from build123d import *

# Parameters (mm, degrees)
F2_R     = 2.6
F3_DEPTH = 6
F4_R     = 4
F5_DEPTH = 28.401


with BuildPart() as f1:
    # F0 (on Front) → F1 (revolve)
    with BuildSketch(Plane.XZ):
        Polygon((48.080009, 8), (48.080009, 18.5), (21.681081, 18.262167), (21.681081, 28.4), (15.681081, 28.4), (15.681081, 8), align=None)
    revolve(axis=Axis((22.226226, 0, 0), (-1, 0, 0)))

    # F2 (on face) → F3 (cut)
    with BuildSketch(Plane.YZ.offset(21.681081)):
        with Locations((-23.400001, 0)):
            Circle(F2_R)
        with Locations((-11.7, -20.264995)):
            Circle(F2_R)
        with Locations((11.7, -20.264995)):
            Circle(F2_R)
        with Locations((23.400001, 0)):
            Circle(F2_R)
        with Locations((11.7, 20.264995)):
            Circle(F2_R)
        with Locations((-11.7, 20.264995)):
            Circle(F2_R)
    extrude(amount=-F3_DEPTH, mode=Mode.SUBTRACT)

    # F4 (on Front) → F5 (cut, through all)
    with BuildSketch(Plane.XZ):
        with Locations((37.880009, 0)):
            Circle(F4_R)
    extrude(amount=-F5_DEPTH, mode=Mode.SUBTRACT)


solid = f1.part
Verification items for the finished model (mm, model axes). A direction names the side the tool comes from. Coordinates: 2 decimals unless noted, no trailing zeros. Write each loop counter-clockwise with the first axis right and the second up, starting at its lowest first coordinate (ties: lowest second). Pieces come first, ordered by that corner, then holes. Notation, with made-up numbers: (70, 86.25) -> (85, 86.25) arc R18 cw to (85, 97.25) -> close; hole circle Ø8 at (-37, 88.5). An arc over 180 degrees is marked (long way). One line per item, written item: value. Start each with the question number.
Q1. Cross-section at D-D on z = -24. Enter the section's corners in (x, y).
Q2. Mould release check, pull along Z, two halves, no side actions. Record for faces 4 (the cylindrical face through (18.639, 28.158, -3.697)), 5 (the flat face through (21.681, 0, -19)), 6 (the cylindrical face through (18.723, -12.038, -17.687)): pulls with the +Z half, pulls with the -Z half, needs draft (parallel to the pull), parting line crosses it, or undercut.
Q3. Cross-section at A-A on y = -23.5. Enter the section's corners in (x, z).
Q4. Cross-section at B-B on y = 11.7. State how many separate pieces and enclosed holes the cut face has, and give its area (3 significant figures).
Q5. Access from +Z, -Z, +X, -X, +Y, -Y to the whole of each face (thin tool, end or side, straight path). Record for faces 1 (the cylindrical face through (41.695, 12.606, 1.201)), 2 (the conical face through (34.696, -17.942, -3.984)), 3 (the cylindrical face through (18.723, 11.362, 22.843)).
Q6. Go/stop test with flat-tipped pins: P1, Ø3, axis at y = 23.4, z = 0, coming from the -X side; P2, Ø8, axis at x = 40.5, z = 15, coming from the -Y side; P3, Ø12, axis at x = 37, y = 18.5, coming from the +Z side; P4, Ø10, axis at x = 33.5, y = 17, coming from the -Z side. Record where each tip stops, or that it passes through.
Q7. Thickness scan on L1, parallel to X at y = 10.75, z = 0; L2, parallel to X at y = 23.5, z = 3.5; L3, parallel to Y at x = 18, z = 0.5. Record the ranges inside material, lowest first. Write a range as from..to.
Q8. Cross-section at C-C on x = 28. Enter the section's corners in (y, z), and give its area (3 significant figures).
Checked values:
1. outline: (15.68, -15.18) -> (21.68, -15.18) -> (21.68, 15.18) -> (15.68, 15.18) -> close
2. face 4: parting line crosses it
2. face 5: needs draft
2. face 6: undercut
3. outline: (15.68, -15.95) -> (21.68, -15.95) -> (21.68, -2.6) -> (15.68, -2.6) -> close; (15.68, 2.6) -> (21.68, 2.6) -> (21.68, 15.95) -> (15.68, 15.95) -> close
4. separate pieces: 3
4. enclosed holes: 1
4. area: 946 mm²
5. face 1: +Y
5. face 2: none
5. face 3: +X, -X
6. P1: passes through
6. P2: stops at y = -14.79
6. P3: stops at z = 13.5
6. P4: stops at z = -13.91
7. L1: x = 15.68..33.88, 41.88..48.08
7. L2: x = 15.68..21.68
7. L3: y = -28.4..-25.95, -20.85..-7.98, 7.98..20.85, 25.95..28.4
8. outline: circle Ø36.64 at (0, 0); hole circle Ø16 at (0, 0)
8. area: 853 mm²
